from build123d import *

# Parameters (mm, degrees)
F0_R     = 1.25
F0_W     = 50
F0_H     = 5
F0_W_2   = 15
F1_DEPTH = 1.5
F0_H_2   = 6.5
F2_DEPTH = 10.5
F0_R_2   = 0.4
F3_DEPTH = 3.6
F4_DEPTH = 10.2
F5_DEPTH = 5


with BuildPart() as f1:
    # F0 (on Front) → F1 (new body)
    with BuildSketch(Plane.XZ):
        with BuildLine():
            Line((38.7267845055, 24.8567230371), (38.7267845055, 25.6081590384))
            ThreePointArc((38.7267845055, 25.6081590384), (37.8486126129, 27.7289714965), (35.7282208505, 28.6081586945))
            Line((35.7282208505, 28.6081586945), (-22.9717791495, 28.6362631804))
            ThreePointArc((-22.9717791495, 28.6362631804), (-25.0940279526, 27.7580916317), (-25.9732154945, 25.6362635243))
            Line((-25.9732154945, 25.6362635243), (-25.9732154945, 21.3067230371))
            Line((-25.9732154945, 21.3067230371), (-19.4732154945, 21.3067230371))
            Line((-19.4732154945, 21.3067230371), (-19.4732154945, -20.3932769629))
            Line((-19.4732154945, -20.3932769629), (-25.9732154945, -20.3932769629))
            Line((-25.9732154945, -20.3932769629), (-25.9732154945, -24.3932769629))
            ThreePointArc((-25.9732154945, -24.3932769629), (-25.094535838, -26.5145973065), (-22.9732154945, -27.3932769629))
            Line((-22.9732154945, -27.3932769629), (-18.2732154945, -27.3932769629))
            Line((-18.2732154945, -27.3932769629), (-18.2732154945, -20.8932769629))
            Line((-18.2732154945, -20.8932769629), (31.7267845055, -20.8932769629))
            Line((31.7267845055, -20.8932769629), (31.7267845055, -27.3932769629))
            Line((31.7267845055, -27.3932769629), (35.4767845055, -27.3932769629))
            ThreePointArc((35.4767845055, -27.3932769629), (37.7748815444, -26.4413740018), (38.7267845055, -24.1432769629))
            Line((38.7267845055, -24.1432769629), (38.7267845055, 24.8567230371))
        make_face()
        with Locations((-22.7232154945, -24.1432769629)):
            Circle(F0_R, mode=Mode.SUBTRACT)
        Polygon((-3.7732154945, -9.8932769629), (-3.7732154945, -8.3932769629), (8.1467845055, -8.3932769629), (9.2267845055, -8.3932769629), (9.2267845055, -9.8932769629), (8.1467845055, -9.8932769629), (7.0267845055, -9.8932769629), (4.8667845055, -9.8932769629), (2.7067845055, -9.8932769629), (0.5467845055, -9.8932769629), (-1.6132154945, -9.8932769629), align=None, mode=Mode.SUBTRACT)
        with Locations((35.4767845055, -24.3807190031)):
            Circle(F0_R, mode=Mode.SUBTRACT)
        with Locations((-22.7232154945, 24.8862631804)):
            Circle(F0_R, mode=Mode.SUBTRACT)
        with Locations((5.9267845055, 24.7324910254)):
            Rectangle(F0_W, F0_H, mode=Mode.SUBTRACT)
        with Locations((27.7267845055, 12.1094132859)):
            Rectangle(F0_W_2, F0_H, mode=Mode.SUBTRACT)
        with Locations((35.4767845055, 24.8567230371)):
            Circle(F0_R, mode=Mode.SUBTRACT)
    extrude(amount=F1_DEPTH)

    # F0 (on Front) → F2 (join)
    with BuildSketch(Plane.XZ):
        Polygon((-19.4732154945, 21.3067230371), (-25.9732154945, 21.3067230371), (-25.9732154945, 8.8067230371), (-25.9732154945, -20.3932769629), (-19.4732154945, -20.3932769629), align=None)
        with Locations((6.7267845055, -24.1432769629)):
            Rectangle(F0_W, F0_H_2)
    extrude(amount=F2_DEPTH)

    # F0 (on Front) → F3 (join)
    with BuildSketch(Plane.XZ):
        with BuildLine():
            Line((8.1467845055, -8.3932769629), (-3.7732154945, -8.3932769629))
            Line((-3.7732154945, -8.3932769629), (-3.7732154945, -9.8932769629))
            Line((-3.7732154945, -9.8932769629), (-1.6132154945, -9.8932769629))
            Line((-1.6132154945, -9.8932769629), (0.5467845055, -9.8932769629))
            Line((0.5467845055, -9.8932769629), (2.7067845055, -9.8932769629))
            Line((2.7067845055, -9.8932769629), (4.8667845055, -9.8932769629))
            Line((4.8667845055, -9.8932769629), (7.0267845055, -9.8932769629))
            Line((7.0267845055, -9.8932769629), (8.1467845055, -9.8932769629))
            Line((8.1467845055, -9.8932769629), (8.1467845055, -9.5432769629))
            ThreePointArc((8.1467845055, -9.5432769629), (7.7467845055, -9.1432769629), (8.1467845055, -8.7432769629))
            Line((8.1467845055, -8.7432769629), (8.1467845055, -8.3932769629))
        make_face()
        with Locations((-2.6932154945, -9.1432769629)):
            Circle(F0_R_2, mode=Mode.SUBTRACT)
        with Locations((-0.5332154945, -9.1432769629)):
            Circle(F0_R_2, mode=Mode.SUBTRACT)
        with Locations((1.6267845055, -9.1432769629)):
            Circle(F0_R_2, mode=Mode.SUBTRACT)
        with Locations((3.7867845055, -9.1432769629)):
            Circle(F0_R_2, mode=Mode.SUBTRACT)
        with Locations((5.9467845055, -9.1432769629)):
            Circle(F0_R_2, mode=Mode.SUBTRACT)
        with BuildLine():
            Line((9.2267845055, -8.3932769629), (8.1467845055, -8.3932769629))
            Line((8.1467845055, -8.3932769629), (8.1467845055, -8.7432769629))
            ThreePointArc((8.1467845055, -8.7432769629), (8.429627218, -8.8604342504), (8.5467845055, -9.1432769629))
            ThreePointArc((8.5467845055, -9.1432769629), (8.429627218, -9.4261196754), (8.1467845055, -9.5432769629))
            Line((8.1467845055, -9.5432769629), (8.1467845055, -9.8932769629))
            Line((8.1467845055, -9.8932769629), (9.2267845055, -9.8932769629))
            Line((9.2267845055, -9.8932769629), (9.2267845055, -8.3932769629))
        make_face()
        with Locations((27.7267845055, 12.1094132859)):
            Rectangle(F0_W_2, F0_H)
        with Locations((21.4767845055, 10.8594132859)):
            Circle(F0_R_2, mode=Mode.SUBTRACT)
        with Locations((21.4767845055, 13.3594132859)):
            Circle(F0_R_2, mode=Mode.SUBTRACT)
        with Locations((23.9767845055, 10.8594132859)):
            Circle(F0_R_2, mode=Mode.SUBTRACT)
        with Locations((26.4767845055, 10.8594132859)):
            Circle(F0_R_2, mode=Mode.SUBTRACT)
        with Locations((28.9767845055, 10.8594132859)):
            Circle(F0_R_2, mode=Mode.SUBTRACT)
        with Locations((23.9767845055, 13.3594132859)):
            Circle(F0_R_2, mode=Mode.SUBTRACT)
        with Locations((26.4767845055, 13.3594132859)):
            Circle(F0_R_2, mode=Mode.SUBTRACT)
        with Locations((28.9767845055, 13.3594132859)):
            Circle(F0_R_2, mode=Mode.SUBTRACT)
        with Locations((31.4767845055, 10.8594132859)):
            Circle(F0_R_2, mode=Mode.SUBTRACT)
        with Locations((33.9767845055, 10.8594132859)):
            Circle(F0_R_2, mode=Mode.SUBTRACT)
        with Locations((31.4767845055, 13.3594132859)):
            Circle(F0_R_2, mode=Mode.SUBTRACT)
        with Locations((33.9767845055, 13.3594132859)):
            Circle(F0_R_2, mode=Mode.SUBTRACT)
    extrude(amount=F3_DEPTH)

    # F0 (on Front) → F4 (join)
    with BuildSketch(Plane.XZ):
        with Locations((21.4767845055, 13.3594132859)):
            Circle(F0_R_2)
        with Locations((23.9767845055, 13.3594132859)):
            Circle(F0_R_2)
        with Locations((26.4767845055, 13.3594132859)):
            Circle(F0_R_2)
        with Locations((28.9767845055, 13.3594132859)):
            Circle(F0_R_2)
        with Locations((31.4767845055, 13.3594132859)):
            Circle(F0_R_2)
        with Locations((33.9767845055, 13.3594132859)):
            Circle(F0_R_2)
        with Locations((21.4767845055, 10.8594132859)):
            Circle(F0_R_2)
        with Locations((23.9767845055, 10.8594132859)):
            Circle(F0_R_2)
        with Locations((26.4767845055, 10.8594132859)):
            Circle(F0_R_2)
        with Locations((28.9767845055, 10.8594132859)):
            Circle(F0_R_2)
        with Locations((31.4767845055, 10.8594132859)):
            Circle(F0_R_2)
        with Locations((33.9767845055, 10.8594132859)):
            Circle(F0_R_2)
        with Locations((-2.6932154945, -9.1432769629)):
            Circle(F0_R_2)
        with Locations((-0.5332154945, -9.1432769629)):
            Circle(F0_R_2)
        with Locations((1.6267845055, -9.1432769629)):
            Circle(F0_R_2)
        with Locations((3.7867845055, -9.1432769629)):
            Circle(F0_R_2)
        with Locations((5.9467845055, -9.1432769629)):
            Circle(F0_R_2)
        with BuildLine():
            ThreePointArc((8.5467845055, -9.1432769629), (8.429627218, -8.8604342504), (8.1467845055, -8.7432769629))
            Line((8.1467845055, -8.7432769629), (8.1467845055, -9.5432769629))
            ThreePointArc((8.1467845055, -9.5432769629), (8.429627218, -9.4261196754), (8.5467845055, -9.1432769629))
        make_face()
        with BuildLine():
            Line((8.1467845055, -9.5432769629), (8.1467845055, -8.7432769629))
            ThreePointArc((8.1467845055, -8.7432769629), (7.7467845055, -9.1432769629), (8.1467845055, -9.5432769629))
        make_face()
    extrude(amount=F4_DEPTH)

    # F0 (on Front) → F5 (join)
    with BuildSketch(Plane.XZ):
        with Locations((5.9267845055, 24.7324910254)):
            Rectangle(F0_W, F0_H)
    extrude(amount=F5_DEPTH)


solid = f1.part
Read the model definition and answer for the solid it produces. Units are mm, in the model's axes. A direction names the side the tool comes from. Give positions to 0.01 mm unless a question says otherwise; leave off trailing zeros. Write each loop counter-clockwise with the first axis right and the second up, starting at its lowest first coordinate (ties: lowest second). Pieces come first, ordered by that corner, then holes. Notation, with made-up numbers: (-32, 48.5) -> (4, 48.5) arc R21 cw to (4, 66.5) -> close; hole circle Ø8 at (-17.5, -28.75). An arc over 180 degrees is marked (long way). Answer as a JSON object with one key per item and string values. Group by question number.
1) Each of these flat-tipped pins is pushed along its axis until it touches: P1, Ø0.6, axis at x = -3, z = -9, coming from the -Y side; P2, Ø6, axis at x = 22, z = -8.5, coming from the -Y side; P3, Ø1.2, axis at y = -2.5, z = -9.5, coming from the +X side. Where does it stop, or does it pass through?
2) Consider L1, parallel to Z at x = 24, y = -3; L2, parallel to Z at x = 21.5, y = -7; L3, parallel to Z at x = 23.5, y = -3.75. Determine where each line is inside the solid, lowest interval first. Write a range as from..to.
3) The mould has two halves that part along X. Classify faces 6 (the flat face through (30.927, -3, 25)), 7 (the flat face through (28, -3, 9.609)), 8 (the cylindrical face through (-21.569, -0.74, 24.408)): +X half, -X half, draft (parallel to the pull), parting line (faces both ways), or undercut.
4) Find section C-C (x = 10.5). Write down the section's boundary in (y, z).
5) Find section D-D (z = -2.5). Write down the section's boundary in (x, y).
6) Find section A-A (z = 12). Write down the section's boundary in (x, y), and give its area (3 significant figures).
7) A tool of negligible diameter and unlimited length cuts with its end or side. For faces 1 (the flat face through (6, -3, 22.232)), 2 (the flat face through (-19.473, -6, 0)), 3 (the flat face through (-18.273, -6, -24)), 4 (the flat face through (-3.773, -3, -9)), 5 (the flat face through (3, -3, -8.393)), from which of +Z, -Z, +X, -X, +Y, -Y can it reach the whole face along a straight path? Write none if from no direction.
8) Find section B-B (y = -6.75). Count the separate pieces of the cut face and the enclosed holes in it, and give its area (3 significant figures).
Values follow:
{
 "1": {"P1": "stops at y = -10.2", "P2": "stops at y = -1.5", "P3": "stops at x = 9.23"},
 "2": {"L1": "z = -27.39..-20.89, 9.61..14.61, 22.23..27.23", "L2": "z = -27.39..-20.89, 10.46..11.26, 12.96..13.76", "L3": "z = -27.39..-20.89, 22.23..27.23"},
 "3": {"face 6": "+X half", "face 7": "draft", "face 8": "undercut"},
 "4": {"outline": "(-10.5, -27.39) -> (0, -27.39) -> (0, 28.62) -> (-1.5, 28.62) -> (-1.5, 27.23) -> (-5, 27.23) -> (-5, 22.23) -> (-1.5, 22.23) -> (-1.5, -20.89) -> (-10.5, -20.89) -> close"},
 "5": {"outline": "(-25.97, -10.5) -> (-19.47, -10.5) -> (-19.47, -1.5) -> (38.73, -1.5) -> (38.73, 0) -> (-25.97, 0) -> close"},
 "6": {"outline": "(-25.97, -10.5) -> (-19.47, -10.5) -> (-19.47, -1.5) -> (20.23, -1.5) -> (20.23, -3.6) -> (35.23, -3.6) -> (35.23, -1.5) -> (38.73, -1.5) -> (38.73, 0) -> (-25.97, 0) -> close", "area": "187 mm2"},
 "7": {"face 1": "+X, -X, -Y", "face 2": "+Z, -Z, -Y", "face 3": "-Z, -X, -Y", "face 4": "-Y", "face 5": "+X, -Y"},
 "8": {"separate pieces": "20", "enclosed holes": "0", "area": "605 mm2"}
}
